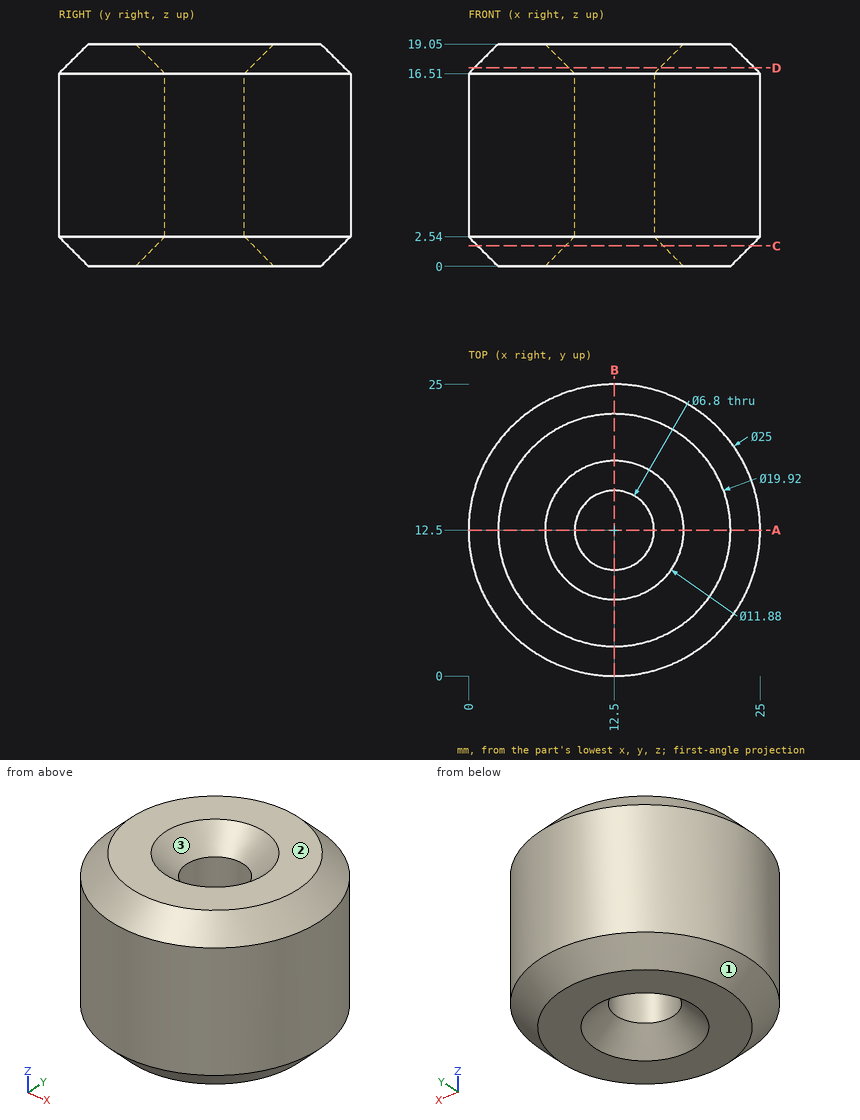
Verification items for this drawing (mm, ordinates from the low corner). Coordinates: 2 decimals unless noted, no trailing zeros. Order: outer loops, then holes, each group sorted by start corner. A loop starts at its lowest first (then second) coordinate and runs counter-clockwise, first axis right, second up. Notation, with made-up numbers: (11.25, 25.5) - (48.25, 25.5) arc R17 ccw to (48.25, 31.5) - close; hole circle Ø9 at (53.5, -24). An arc over 180 degrees is marked (long way). Use one line per item in the form item = value.
1. Draft check along Y on the marked faces 1, 2 and 3. Enter one of: pulls with the +Y half, pulls with the -Y half, needs draft (parallel to the pull), parting line crosses it, or undercut.
Here are the results:
face_1 = parting line crosses it
face_2 = needs draft
face_3 = undercut
2. Section check C-C (z = 1.75). Record the boundary of the cut face in (x, y).
Here are the results:
outline = circle Ø23.42 at (12.5, 12.5); hole circle Ø8.38 at (12.5, 12.5)
3. Section check D-D (z = 17). Record the boundary of the cut face in (x, y).
Here are the results:
outline = circle Ø24.02 at (12.5, 12.5); hole circle Ø7.78 at (12.5, 12.5)
4. Scan lines: line 1 (Y direction, x = 12.5, z = 8); line 2 (X direction, y = 14, z = 8.5); line 3 (X direction, y = 13.25, z = 9.5). Record each from-to range of solid material in increasing order.
Here are the results:
line_1 = 0 to 9.1, 15.9 to 25
line_2 = 0.09 to 9.45, 15.55 to 24.91
line_3 = 0.02 to 9.18, 15.82 to 24.98
5. Gauge pin test, flat ends, axial feed: pin 1 (2 mm diameter, centred on x = 4, y = 18.5, fed in from -Z); pin 2 (5 mm diameter, centred on y = 4.5, z = 4, fed in from -X) (3 decimals); pin 3 (1.5 mm diameter, centred on y = 16.5, z = 2.5, fed in from +X); pin 4 (6 mm diameter, centred on y = 17.5, z = 13, fed in from -X). Record the tip position at first contact, or that the pin passes through.
Here are the results:
pin_1 = 0
pin_2 = 1.275
pin_3 = 24.57
pin_4 = 0.16
6. Section check A-A (y = 12.5). Record the boundary of the cut face in (x, z).
Here are the results:
outline = (0, 2.54) - (2.54, 0) - (6.56, 0) - (9.1, 2.54) - (9.1, 16.51) - (6.56, 19.05) - (2.54, 19.05) - (0, 16.51) - close; (15.9, 2.54) - (18.44, 0) - (22.46, 0) - (25, 2.54) - (25, 16.51) - (22.46, 19.05) - (18.44, 19.05) - (15.9, 16.51) - close
